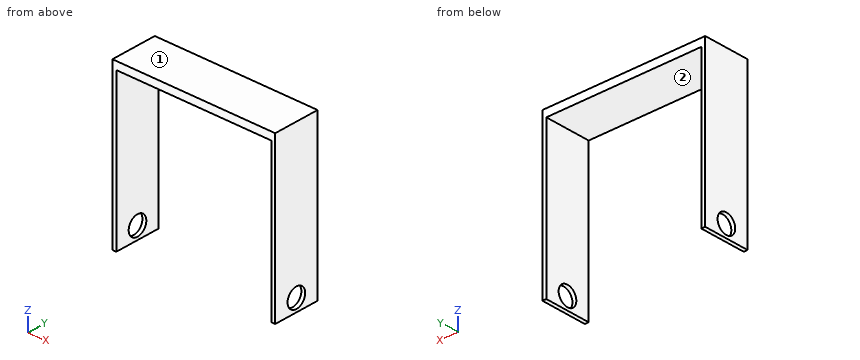
```python
from build123d import *

# Parameters (mm, degrees)
F0_W     = 106.68
F0_H     = 106.68
F1_DEPTH = 30.48
F2_W     = 101.6
F2_H     = 101.6
F3_DEPTH = 30.48
F4_R     = 6.35
F5_DEPTH = 106.68


with BuildPart() as f1:
    # F0 (on Front) → F1 (new body)
    with BuildSketch(Plane.XZ):
        with Locations((53.34, 53.34)):
            Rectangle(F0_W, F0_H)
    extrude(amount=F1_DEPTH)

    # F2 (on face) → F3 (cut)
    with BuildSketch(Plane.XZ.offset(30.48)):
        with Locations((53.34, 50.8)):
            Rectangle(F2_W, F2_H)
    extrude(amount=-F3_DEPTH, mode=Mode.SUBTRACT)

    # F4 (on face) → F5 (cut)
    with BuildSketch(Plane.YZ.offset(106.68)):
        with Locations((-15.24, 8.207626)):
            Circle(F4_R)
    extrude(amount=-F5_DEPTH, mode=Mode.SUBTRACT)


solid = f1.part
```
Design review of the part built by this model. Coordinates are the model's own, in mm. Face numbers are marked on the shaded views. A direction names the side the tool comes from. Give positions to 0.01 mm unless a question says otherwise; leave off trailing zeros. Write each loop counter-clockwise with the first axis right and the second up, starting at its lowest first coordinate (ties: lowest second). Pieces come first, ordered by that corner, then holes.
(1) Add section B-B (y = -15.24). Give the boundary of the cut face in (x, z).
Checked values:
outline: (0, 0) - (2.54, 0) - (2.54, 1.86) - (0, 1.86) - close; (0, 14.56) - (2.54, 14.56) - (2.54, 101.6) - (104.14, 101.6) - (104.14, 14.56) - (106.68, 14.56) - (106.68, 106.68) - (0, 106.68) - close; (104.14, 0) - (106.68, 0) - (106.68, 1.86) - (104.14, 1.86) - close
(2) Add section A-A (z = 70.5). Give the boundary of the cut face in (x, y), and give its area (3 significant figures).
Checked values:
outline: (0, -30.48) - (2.54, -30.48) - (2.54, 0) - (0, 0) - close; (104.14, -30.48) - (106.68, -30.48) - (106.68, 0) - (104.14, 0) - close
area: 155 mm2
(3) Add section C-C (x = 82). Give the boundary of the cut face in (y, z), and give its area (3 significant figures).
Checked values:
outline: (-30.48, 101.6) - (0, 101.6) - (0, 106.68) - (-30.48, 106.68) - close
area: 155 mm2
(4) Wall thickness on line 1 along X through (y, z) = (-23.5, 49); line 2 along Z through (x, y) = (105, -15); line 3 along Z through (x, y) = (24.5, -24): over which ranges is each line inside the solid? List them lowest first.
Checked values:
line 1: x = 0 to 2.54, 104.14 to 106.68
line 2: z = 0 to 1.86, 14.55 to 106.68
line 3: z = 101.6 to 106.68
(5) Clearance check with a flat-ended pin moving along its axis: pin 1 Ø1 at (x, y) = (51, -18) entering from -Z. State where the tip first meets the part, or that it passes through.
Checked values:
pin 1: stops at z = 101.6
(6) Tool access review of the marked faces 1 and 2: name each direction out of +Z, -Z, +X, -X, +Y, -Y from which nothing blocks a thin tool from reaching the whole face with its end or side.
Checked values:
face 1: +Z, +X, -X, +Y, -Y
face 2: -Z, +Y, -Y
